For this review, take the finished solid that the model builds, in its own axes (mm). Face numbers are marked on the shaded views. A direction names the side the tool comes from. Coordinates: 2 decimals unless noted, no trailing zeros. Order: outer loops, then holes, each group sorted by start corner. A loop starts at its lowest first (then second) coordinate and runs counter-clockwise, first axis right, second up. Notation, with made-up numbers: (54.5, 15) -> (65.5, 15) arc R37 cw to (65.5, 51) -> close; hole circle Ø9 at (54.5, 60). An arc over 180 degrees is marked (long way). Return JSON: item names as keys, results as strings. Group by question number.
Item 1: Take a section at B-B (x = -5.5). Write out the cut boundary in (y, z) (3 decimals), then the cut area to 3 significant figures.
Item 2: Take a section at C-C (z = 1.25). Write out the cut boundary in (x, y).
Item 3: Insertion check: pin 1 (2 mm diameter, centred on x = -5, z = 10.5, fed in from -Y); pin 2 (1.5 mm diameter, centred on y = 9, z = 0.5, fed in from -X); pin 3 (1.5 mm diameter, centred on x = -3.5, z = 2, fed in from +Y). Each pin has a flat end and moves straight along its axis. Give the tip position at first contact, or say it passes through.
Item 4: Machinability: for the marked faces 4 and 5, which of the approach directions +Z, -Z, +X, -X, +Y, -Y give a long, thin tool a straight path to every point of the face, cutting with its end or side? Answer none if there is none.
Item 5: Draft analysis for pull direction Z (two halves, no side actions). For the marked faces 1, 2 and 3, state which applies: +Z half, -Z half, draft (parallel to the pull), parting line (faces both ways), or undercut.
Item 6: Take a section at D-D (x = -12.5). Write out the cut boundary in (y, z) (3 decimals).
Item 7: For line 1 along Z through (x, y) = (-6, 8.75); line 2 along Z through (x, y) = (-19, 3.75); line 3 along Y through (x, z) = (-21, -0.25), list the stretches that pass through material, from the lowest coordinate up.
Item 8: Take a section at A-A (y = 6). Write out the cut boundary in (x, z), then the cut area to 3 significant figures.
```python
from build123d import *

# Parameters (mm, degrees)
BOSS_EXTRUDE2_DEPTH = 3
BOSS_EXTRUDE3_DEPTH = 7.5
BOSS_EXTRUDE4_START = 2
BOSS_EXTRUDE4_DEPTH = 2
SKETCH5_R           = 2.4
BOSS_EXTRUDE5_DEPTH = 8


with BuildPart() as part:
    # Sketch1 → Boss-Extrude2 (new body)
    with BuildSketch(Plane(origin=(0, 0, 0), x_dir=(0, 1, 0), z_dir=(0, 0, 1))):
        with BuildLine():
            Line((0, 0), (1.5, 0))
            Line((1.5, 0), (1.5, 5))
            Line((1.5, 5), (3, 15))
            ThreePointArc((3, 15), (6, 18), (9, 15))
            Line((9, 15), (10.5, 5))
            Line((10.5, 5), (10.5, 0))
            Line((10.5, 0), (12, 0))
            Line((12, 0), (10.5, 21))
            ThreePointArc((10.5, 21), (6, 25.5), (1.5, 21))
            Line((1.5, 21), (0, 0))
        make_face()
    extrude(amount=BOSS_EXTRUDE2_DEPTH)

    # Sketch3 → Boss-Extrude3 (add)
    with BuildSketch(Plane.XY.offset(3)):
        with BuildLine():
            Line((0, 0), (0, 12))
            Line((0, 12), (-21, 10.5))
            ThreePointArc((-21, 10.5), (-25.5, 6), (-21, 1.5))
            Line((-21, 1.5), (0, 0))
        make_face()
    extrude(amount=BOSS_EXTRUDE3_DEPTH)

    # Sketch4 → Boss-Extrude4 (add)
    with BuildSketch(Plane(origin=(0, 0, 0), x_dir=(1, 0, 0), z_dir=(0, 0, -1)).offset(BOSS_EXTRUDE4_START)):
        with BuildLine():
            Line((0, 0), (0, -12))
            Line((0, -12), (-21, -10.5))
            ThreePointArc((-21, -10.5), (-25.5, -6), (-21, -1.5))
            Line((-21, -1.5), (0, 0))
        make_face()
    extrude(amount=-BOSS_EXTRUDE4_DEPTH)

    # Sketch5 → Boss-Extrude5 (add)
    with BuildSketch(Plane.XY.offset(10.5)):
        with Locations((-21, 6)):
            Circle(SKETCH5_R)
    extrude(amount=BOSS_EXTRUDE5_DEPTH)


solid = part.part
```
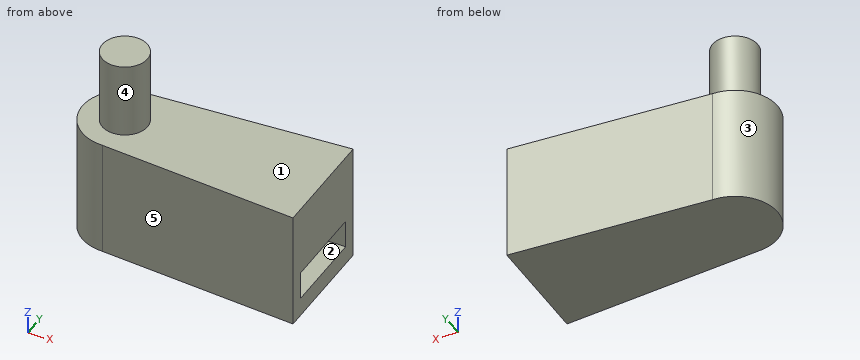
Findings below:
{
 "1": {"outline": "(0.393, -2) -> (11.607, -2) -> (11.607, 10.5) -> (0.393, 10.5) -> close; hole (1.575, 0) -> (10.425, 0) -> (10.425, 3) -> (1.575, 3) -> close", "area": "114 mm2"},
 "2": {"outline": "(-21, 1.5) -> (0, 0) -> (0, 1.5) -> (-5, 1.5) -> (-15, 3) arc R3 cw to (-15, 9) -> (-5, 10.5) -> (0, 10.5) -> (0, 12) -> (-21, 10.5) arc R4.5 ccw to start"},
 "3": {"pin 1": "stops at y = 0.29", "pin 2": "stops at x = -24.9", "pin 3": "stops at y = 11.8"},
 "4": {"face 4": "+Z", "face 5": "+Z, -Z, -X, -Y"},
 "5": {"face 1": "+Z half", "face 2": "undercut", "face 3": "draft"},
 "6": {"outline": "(0.893, -2) -> (11.107, -2) -> (11.107, 10.5) -> (0.893, 10.5) -> close; hole (2.625, 0) -> (9.375, 0) -> (9.375, 3) -> (2.625, 3) -> close"},
 "7": {"line 1": "z = -2 to 0, 3 to 10.5", "line 2": "z = -2 to 10.5", "line 3": "y = 1.5 to 10.5"},
 "8": {"outline": "(-25.5, -2) -> (0, -2) -> (0, 0) -> (-18, 0) -> (-18, 3) -> (0, 3) -> (0, 10.5) -> (-18.6, 10.5) -> (-18.6, 18.5) -> (-23.4, 18.5) -> (-23.4, 10.5) -> (-25.5, 10.5) -> close", "area": "303 mm2"}
}
